CAD build for the part. Positions are in the model's coordinates, mm. A direction names the side the tool comes from. Give positions to 0.01 mm unless a question says otherwise; leave off trailing zeros. Loops run counter-clockwise (first coordinate to the right, second up) from the corner with the lowest first, then second, coordinate; pieces in that order, holes last. Notation, with made-up numbers: (66, 75) - (85, 75) arc R18 ccw to (85, 108) - close; hole circle Ø4 at (86.25, -11.5). An arc over 180 degrees is marked (long way). Return JSON: item names as keys, results as strings.
from build123d import *

# Parameters (mm, degrees)
BOSS_EXTRUDE1_DEPTH = 5
CUT_EXTRUDE1_DEPTH  = 5


with BuildPart() as part:
    # Sketch2 → Boss-Extrude1 (new body)
    with BuildSketch(Plane(origin=(0, 0, 0), x_dir=(1, 0, 0), z_dir=(0, 1, 0))):
        Polygon((-15.5, -26), (15.5, -26), (26, -15.5), (26, 15.5), (15.5, 26), (-15.5, 26), (-26, 15.5), (-26, -15.5), align=None)
    extrude(amount=BOSS_EXTRUDE1_DEPTH)

    # Sketch3 → Cut-Extrude1 (cut)
    with BuildSketch(Plane(origin=(0, 5, 0), x_dir=(1, 0, 0), z_dir=(0, 1, 0))):
        Polygon((-21.1, -15.6), (-21.1, 15.6), (-15.6, 21.1), (15.6, 21.1), (21.1, 15.6), (21.1, -15.6), (15.6, -21.1), (-15.6, -21.1), align=None)
    extrude(amount=-CUT_EXTRUDE1_DEPTH, mode=Mode.SUBTRACT)


solid = part.part
1. Cut at A-A, the plane z = 18. Write the cut outline in (x, y).
Values follow:
{"outline": "(-23.5, 0) - (-18.7, 0) - (-18.7, 5) - (-23.5, 5) - close; (18.7, 0) - (23.5, 0) - (23.5, 5) - (18.7, 5) - close"}
2. Which spindle directions (+Z, -Z, +X, -X, +Y, -Y) get a long thin tool onto all of the face, cutting with end or side? Do faces 1 (the face through (-21.3, 5, -0.1)), 2 (the face through (0, 3, -21.1)). Say none if no direction does.
Values follow:
{"face 1": "+Z, -Z, +X, -X, +Y", "face 2": "+Y, -Y"}
3. Drill centre lines: probe 1 along Z at (x, y) = (-11, 1.4); probe 2 along X at (y, z) = (2.45, 18). Where is each one in solid material? Low to high.
Values follow:
{"probe 1": "z = -26 to -21.1, 21.1 to 26", "probe 2": "x = -23.5 to -18.7, 18.7 to 23.5"}
4. Pull direction X, two halves, no side cores. Call faces 3 (the face through (-20.7, 2.5, -20.8)), 4 (the face through (0, 3, 21.1)), 5 (the face through (18.4, 2.5, 18.3)), 6 (the face through (26, 2, 0)): +X half, -X half, draft (parallel to the pull), parting line (faces both ways), or undercut.
Values follow:
{"face 3": "-X half", "face 4": "undercut", "face 5": "undercut", "face 6": "+X half"}
5. Cut at C-C, the plane y = 4.2. Write the cut outline in (x, z).
Values follow:
{"outline": "(-26, -15.5) - (-15.5, -26) - (15.5, -26) - (26, -15.5) - (26, 15.5) - (15.5, 26) - (-15.5, 26) - (-26, 15.5) - close; hole (-21.1, -15.6) - (-15.6, -21.1) - (15.6, -21.1) - (21.1, -15.6) - (21.1, 15.6) - (15.6, 21.1) - (-15.6, 21.1) - (-21.1, 15.6) - close"}
6. Cut at B-B, the plane x = 12. Write the cut outline in (y, z), plus the area to 3 significant figures.
Values follow:
{"outline": "(0, -26) - (5, -26) - (5, -21.1) - (0, -21.1) - close; (0, 21.1) - (5, 21.1) - (5, 26) - (0, 26) - close", "area": "49.0 mm²"}
